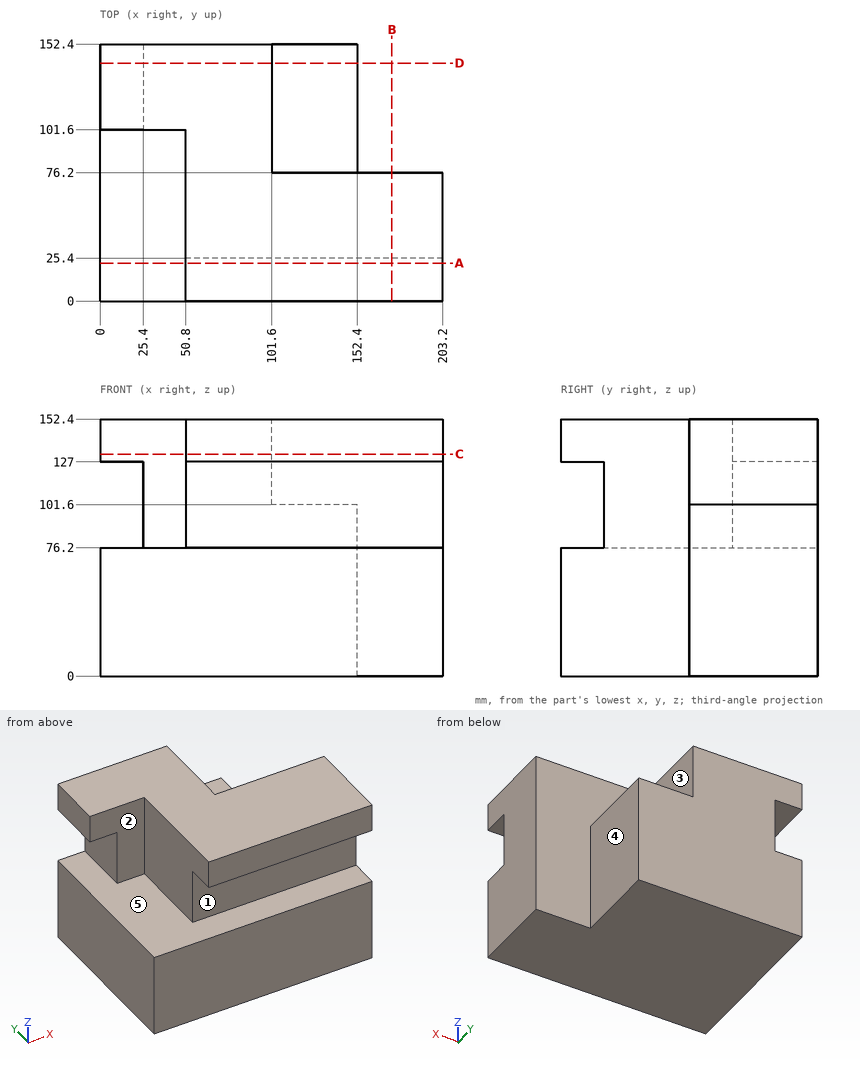
The drawing under review shows one solid part. Ordinate dimensions are in mm from its lowest x, y, z. A direction names the side the tool comes from. Round coordinates to 2 decimals unless told otherwise and drop trailing zeros. Write each loop counter-clockwise with the first axis right and the second up, starting at its lowest first coordinate (ties: lowest second). Pieces come first, ordered by that corner, then holes. Notation, with made-up numbers: M 55,89.5 L 93,89.5 A23 ccw 93,109.5 Z; hole C 55,-12 d10. An arc over 180 degrees is marked long. One line per item, written item: value. Start each with the question number.
(1) We need section C-C (z = 131.5). Give the boundary of the cut face in (x, y), and give its area (3 significant figures).
(2) We need section D-D (y = 141). Give the boundary of the cut face in (x, z), and give its area (3 significant figures).
(3) Wall thickness on line 1 (Y direction, x = 142, z = 91.5); line 2 (Y direction, x = 170, z = 107); line 3 (Z direction, x = 127, y = 119): over which ranges is each line inside the solid? List them lowest first.
(4) We need section A-A (y = 22.5). Give the boundary of the cut face in (x, z).
(5) Insertion check: pin 1 (8 mm diameter, centred on y = 102.5, z = 103, fed in from +X); pin 2 (3 mm diameter, centred on y = 48, z = 94, fed in from -X); pin 3 (10 mm diameter, centred on x = 38, z = 129.5, fed in from -Y). Each pin has a flat end and moves straight along its axis. Give the tip position at first contact, or say it passes through.
(6) Machinability: for the marked faces 1, 2, 3, 4 and 5, which of the approach directions +Z, -Z, +X, -X, +Y, -Y give a long, thin tool a straight path to every point of the face, cutting with its end or side? Answer none if there is none.
(7) We need section B-B (x = 173). Give the boundary of the cut face in (y, z).
Result:
1. outline: M 0,101.6 L 50.8,101.6 L 50.8,0 L 203.2,0 L 203.2,76.2 L 101.6,76.2 L 101.6,152.4 L 0,152.4 Z
1. area: 18,100 mm²
2. outline: M 0,0 L 152.4,0 L 152.4,101.6 L 101.6,101.6 L 101.6,152.4 L 0,152.4 L 0,127 L 25.4,127 L 25.4,76.2 L 0,76.2 Z
2. area: 19,400 mm²
3. line 1: 25.4 to 152.4
3. line 2: 25.4 to 76.2
3. line 3: 0 to 101.6
4. outline: M 0,0 L 203.2,0 L 203.2,76.2 L 0,76.2 Z; M 50.8,127 L 203.2,127 L 203.2,152.4 L 50.8,152.4 Z
5. pin 1: x = 152.4
5. pin 2: x = 50.8
5. pin 3: y = 101.6
6. face 1: +X, -X, -Y
6. face 2: +Z, -X, -Y
6. face 3: +Z, +X, +Y
6. face 4: +Z, -Z, +X, +Y
6. face 5: -X, -Y
7. outline: M 0,0 L 76.2,0 L 76.2,152.4 L 0,152.4 L 0,127 L 25.4,127 L 25.4,76.2 L 0,76.2 Z
